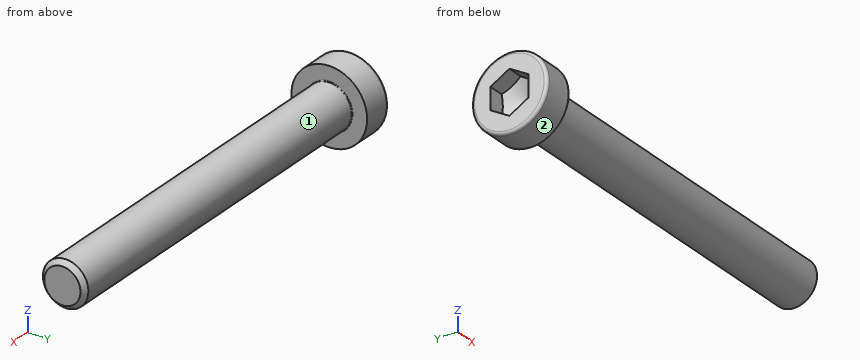
Autodesk Inventor part; units mm, degrees
ref_plane "Work Plane1" through (29, 0, 0) normal (0, -1, 0) x (1, 0, 0)
ref_plane "YZ Plane" through (0, 0, 0) normal (1, 0, 0) x (0, 1, 0)
ref_plane "XZ Plane" through (0, 0, 0) normal (0, 1, 0) x (-1, 0, 0)
sketch "Sketch1" plane through (0, 0, 0) normal (0, 0, 1) x (1, 0, 0)
  line L0 (-0.2433, 0) -> (50, 0)
  line L1 (50, 0) -> (50, 3)
  line L2 (50, 3) -> (26, 3)
  line L3 (26, 3) -> (25.3864, 3)
  line L4 (25.3864, 3) -> (0, 3)
  line L5 (0, 3) -> (0, 5)
  line L6 (0, 5) -> (-4, 5)
  line L7 (-4, 5) -> (-4, 2.8868)
  line L8 (-4, 2.8868) -> (-1.91, 2.8868)
  line L9 (-1.91, 2.8868) -> (-0.2433, 0)
  line L10 (-14.8, 0) -> (60.8, 0)
  line L11 (0, -1) -> (0, 6)
  line L12 (26, 3) -> (0, 3) construction
  dimension "d1" = 24
  dimension "d2" = 0.6136
  dimension "d3" = 4
  dimension "d4" = 2.09
  dimension "d5" = 60
  dimension "d6" = 6
  dimension "d7" = 6
  dimension "d8" = 5.7735
  dimension "d9" = 10
  dimension "d26" = 50
revolve "Body" add sketch "Sketch1" angle 360 about axis through (-0.2433, 0, 0) along (1, 0, 0)
sketch "Sketch2" plane through (-4, 0, 0) normal (-1, 0, 0) x (0, 0, 1)
  circle A0 centre (0, 0) radius 2.8868
  line L0 (0, -7) -> (0, 7)
  line L1 (-7, 0) -> (7, 0)
  line L2 (2.8868, 0) -> (1.4434, -2.5)
  line L3 (1.4434, -2.5) -> (-1.4434, -2.5)
  line L4 (-1.4434, -2.5) -> (-2.8868, 0)
  line L5 (-2.8868, 0) -> (-1.4434, 2.5)
  line L6 (-1.4434, 2.5) -> (1.4434, 2.5)
  line L7 (1.4434, 2.5) -> (2.8868, 0)
extrude "Slot" add sketch "Sketch2" against normal up to next contours L7 A0 | A0 L2 | L6 L0 A0 | A0 L0 L3 | L0 L6 A0 | A0 L3 L0 | L4 A0 | A0 L5
fillet "Fillet1" radius 0.4 1 edges at (-4, -5, 0)
thread "Thread"
chamfer "Chamfer1" distance 0.6135 distance2 0.6135 1 edges at (50, -3, 0) measured on face at (50, -0.7485, -0.2663)
ref_plane "Work Plane1" through (29, 0, 0) normal (0, -1, 0) x (1, 0, 0)
fillet "Fillet2" radius 0.1 1 edges at (0, -3, 0)
equation "\"d1\" = GEL"
equation "\"d3\" = KOH"
equation "\"d4\" = INTI"
equation "\"d6\" = GD"
equation "\"d7\" = BDM"
equation "\"d8\" = 1.1547 * SW"
equation "\"d9\" = KOD"
equation "\"d26\" = NLG"
equation "\"d30\" = R"
equation "\"d17\" = RR"
equation "\"d13\" = GEL"
equation "\"d15\" = -0.5 * SPD + 0.5 * GD"
equation "\"d16\" = GUL"
equation "\"GD\" = NND"
equation "\"NLG\" = 50"
equation "\"GEL\" = 24"
equation "\"KOD\" = 10"
equation "\"KOH\" = 4"
equation "\"INTI\" = 2.09"
equation "\"GAL\" = 0.61345 * PTC"
equation "\"GUL\" = 0.61345 * PTC"
equation "\"BDM\" = NND"
equation "\"SW\" = 5"
equation "\"RR\" = 0.4"
equation "\"SPD\" = NND - 1.2269 * PTC"
equation "\"R\" = 0.1"
equation "\"PHH\" = 0.4"
equation "\"GD1\" = THREADDIA - 1.2269 * PTC"
equation "\"THREADDIA\" = 6"
equation "\"FAWI\" = 45deg"
equation "\"PTC\" = 1"
equation "\"NND\" = 6"
equation "\"FAWI1\" = 30deg"
equation "\"TOA\" = 30deg"
equation "\"E0\" = 1.155 * SW"
properties part number "Unbrako - M6 x 50" material "Steel, Mild"
The model under review builds one solid part; all positions refer to its coordinate system, in mm. Face numbers are marked on the shaded views. A direction names the side the tool comes from. Give positions to 0.01 mm unless a question says otherwise; leave off trailing zeros. Order: outer loops, then holes, each group sorted by start corner. A loop starts at its lowest first (then second) coordinate and runs counter-clockwise, first axis right, second up. Notation, with made-up numbers: M 13.25,20.25 L 60.25,20.25 A24 cw 60.25,53.25 Z; hole C 80,-0.5 d3. An arc over 180 degrees is marked long. Answer in a Markdown table with one row per item. Add a question column.
1. Add section A-A on x = 36. State the section outline as (y, z) points.
2. Machinability: for the marked faces 1 and 2, which of the approach directions +Z, -Z, +X, -X, +Y, -Y give a long, thin tool a straight path to every point of the face, cutting with its end or side? Answer none if there is none.
3. To check wall thickness, follow line 1 along X through (y, z) = (3.25, 0.5); line 2 along X through (y, z) = (0.5, -2); line 3 along Z through (x, y) = (45.5, 0.25). State the ranges of each line that lie inside material, in increasing order.
4. For pin 1 Ø1.2 at (x, z) = (-2.5, -0.5) entering from -Y; pin 2 Ø6 at (x, y) = (15, -1) entering from +Z; pin 3 Ø6 at (x, z) = (20.5, -3.5) entering from -Y; pin 4 Ø6 at (x, y) = (7, -0.5) entering from -Z, all flat-tipped, find the tip position at first contact; note any pin that passes through.
The answers:
| question | item | result |
|---|---|---|
| 1 | outline | C 0,0 d6 |
| 2 | face 1 | +X |
| 2 | face 2 | +X, -X |
| 3 | line 1 | -4 to 0 |
| 3 | line 2 | -1.43 to 50 |
| 3 | line 3 | -2.99 to 2.99 |
| 4 | pin 1 | y = -5 |
| 4 | pin 2 | z = 3 |
| 4 | pin 3 | y = -2.96 |
| 4 | pin 4 | z = -3 |
